Model file for the job. Use its own axes, mm. A direction names the side the tool comes from. Give positions to 0.01 mm unless a question says otherwise; leave off trailing zeros. Loops run counter-clockwise (first coordinate to the right, second up) from the corner with the lowest first, then second, coordinate; pieces in that order, holes last. Notation, with made-up numbers: M 74.25,42.25 L 82.25,42.25 A27 cw 82.25,77.25 Z; hole C 63,9.5 d5. An arc over 180 degrees is marked long. Answer in a Markdown table with one row per item.
```python
from build123d import *

# Parameters (mm, degrees)
BOSS_EXTRUDE1_DEPTH = 1.6
FILLET1_R           = 0.1
SKETCH2_R           = 1
SKETCH2_W           = 3.5
SKETCH2_H           = 8
CUT_EXTRUDE1_DEPTH  = 76.976566532
FILLET2_R           = 0.3


with BuildPart() as part:
    # Sketch1 → Boss-Extrude1 (new body)
    with BuildSketch(Plane(origin=(0, 0, 0), x_dir=(1, 0, 0), z_dir=(0, 1, 0))):
        with BuildLine():
            Line((0, 0), (0, 55.77852758))
            ThreePointArc((0, 55.77852758), (1.60175081, 65.88455922), (6.25, 75))
            ThreePointArc((6.25, 75), (10.68267286, 65.814463025), (12.5, 55.77852758))
            Line((12.5, 55.77852758), (12.5, 0))
            Line((12.5, 0), (0, 0))
        make_face()
    extrude(amount=BOSS_EXTRUDE1_DEPTH)

    # Fillet1
    fillet1_edges = [part.edges().sort_by_distance(p)[0] for p in [
        (6.25, 0.8, -75),
    ]]
    fillet(fillet1_edges, radius=FILLET1_R)

    # Sketch2 → Cut-Extrude1 (cut, through all)
    with BuildSketch(Plane(origin=(0, 1.6, 0), x_dir=(1, 0, 0), z_dir=(0, 1, 0))):
        with Locations(Location((6.5, 4, 0), (0, 0, 270))):
            Circle(SKETCH2_R)
        with Locations((1.75, 4)):
            Rectangle(SKETCH2_W, SKETCH2_H)
    extrude(amount=-CUT_EXTRUDE1_DEPTH, mode=Mode.SUBTRACT)

    # Fillet2
    fillet2_edges = [part.edges().sort_by_distance(p)[0] for p in [
        (0, 0.8, -8),
        (3.5, 0.8, -8),
        (3.5, 0.8, 0),
        (12.5, 0.8, 0),
    ]]
    fillet(fillet2_edges, radius=FILLET2_R)


solid = part.part
```
(1) Saw through at C-C, the plane x = 1.75. Give the cut face in (y, z), and give its area (3 significant figures).
Established:
| item | result |
|---|---|
| outline | M 0,-66.33 L 1.6,-66.33 L 1.6,-8 L 0,-8 Z |
| area | 93.3 mm2 |
(2) Saw through at B-B, the plane z = -61. Give the cut face in (x, y), and give its area (3 significant figures).
Established:
| item | result |
|---|---|
| outline | M 0.42,0 L 11.91,0 L 11.91,1.6 L 0.42,1.6 Z |
| area | 18.4 mm2 |
(3) Wall check: L1, parallel to X at y = 1.3, z = -4; L2, parallel to X at y = 0.1, z = -5.5; L3, parallel to Z at x = 8.5, y = 0.75. Give the ranges that are in metal, low to high.
Established:
| item | result |
|---|---|
| L1 | x = 3.5 to 5.5, 7.5 to 12.5 |
| L2 | x = 3.5 to 12.5 |
| L3 | z = -71.12 to 0 |
(4) Flat gauge pin, fed straight in: P1, Ø0.5, axis at x = 2, y = 0.5, coming from the +Z side. Where does the tip first touch, or does it go through?
Established:
| item | result |
|---|---|
| P1 | stops at z = -8 |
(5) Saw through at A-A, the plane z = -4. Give the cut face in (x, y), and give its area (3 significant figures).
Established:
| item | result |
|---|---|
| outline | M 3.5,0 L 5.5,0 L 5.5,1.6 L 3.5,1.6 Z; M 7.5,0 L 12.5,0 L 12.5,1.6 L 7.5,1.6 Z |
| area | 11.2 mm2 |
(6) Which spindle directions (+Z, -Z, +X, -X, +Y, -Y) get a long thin tool onto all of the face, cutting with end or side? Do faces 5 (the flat face through (2, 1, -8)), 6 (the flat face through (6, 0, -38)). Say none if no direction does.
Established:
| item | result |
|---|---|
| face 5 | +Z, -X, +Y, -Y |
| face 6 | +Z, -Z, +X, -X, -Y |
(7) Mould opens along X. For faces 1 (the flat face through (3.5, 1, -4)), 2 (the cylindrical face through (10.66, 0.79, -65.88)), 3 (the flat face through (6, 1.6, -38)), 4 (the cylindrical face through (7.176, 0.811, -4.737)) say: pulls with the +X half, pulls with the -X half, needs draft (parallel to the pull), parting line crosses it, or undercut.
Established:
| item | result |
|---|---|
| face 1 | pulls with the -X half |
| face 2 | pulls with the +X half |
| face 3 | needs draft |
| face 4 | undercut |
